```python
from build123d import *

# Parameters (mm, degrees)
SKETCH_W            = 9
SKETCH_H            = 10
PAD_DEPTH           = 30
SKETCH001_R         = 1.5
POCKET_DEPTH        = 5.501
POCKET_DEPTH_BACK   = 5.501
LINEARPATTERN_COUNT = 4
LINEARPATTERN_PITCH = 6.666667


with BuildPart() as part:
    # Sketch → Pad (new body)
    with BuildSketch(Plane.XY):
        Polygon((-5.5, 6), (-5.5, -6), (-1, -6), (-1, -16), (1, -16), (1, -6), (5.5, -6), (5.5, 6), align=None)
        Rectangle(SKETCH_W, SKETCH_H, mode=Mode.SUBTRACT)
    extrude(amount=PAD_DEPTH)

    # Sketch001 → Pocket (cut, two sides)
    with BuildSketch(Plane.YZ) as pocket_sk:
        with Locations((-11, 5)):
            Circle(SKETCH001_R)
    pocket = extrude(amount=-POCKET_DEPTH, mode=Mode.SUBTRACT) + extrude(pocket_sk.sketch, amount=POCKET_DEPTH_BACK, mode=Mode.SUBTRACT)

    # LinearPattern: Pocket ×4
    with Locations(*[(0, 0, i * LINEARPATTERN_PITCH) for i in range(1, LINEARPATTERN_COUNT)]):
        add(pocket, mode=Mode.SUBTRACT)


solid = part.part
```
Read the model definition and answer for the solid it produces. Units are mm, in the model's axes. A direction names the side the tool comes from. Round coordinates to 2 decimals unless told otherwise and drop trailing zeros. Write each loop counter-clockwise with the first axis right and the second up, starting at its lowest first coordinate (ties: lowest second). Pieces come first, ordered by that corner, then holes. Notation, with made-up numbers: M 34.5,49 L 41.5,49 A21 ccw 41.5,72 Z; hole C 50,-4.5 d5. An arc over 180 degrees is marked long. One line per item, written item: value.
Q1. Find section D-D on x = 2.75. Write down the section's boundary in (y, z).
Data:
outline: M -6,0 L -5,0 L -5,30 L -6,30 Z; M 5,0 L 6,0 L 6,30 L 5,30 Z
Q2. Find section B-B on y = -11. Write down the section's boundary in (x, z).
Data:
outline: M -1,0 L 1,0 L 1,3.5 L -1,3.5 Z; M -1,6.5 L 1,6.5 L 1,10.17 L -1,10.17 Z; M -1,13.17 L 1,13.17 L 1,16.83 L -1,16.83 Z; M -1,19.83 L 1,19.83 L 1,23.5 L -1,23.5 Z; M -1,26.5 L 1,26.5 L 1,30 L -1,30 Z
Q3. Find section C-C on z = 14.5. Write down the section's boundary in (x, y).
Data:
outline: M -5.5,-6 L -1,-6 L -1,-16 L 1,-16 L 1,-6 L 5.5,-6 L 5.5,6 L -5.5,6 Z; hole M -4.5,-5 L 4.5,-5 L 4.5,5 L -4.5,5 Z
Q4. Which of the six approach directions +Z, -Z, +X, -X, +Y, -Y give full straight-line access (tool end or side, diameter ignored) to faces 4 (the flat face through (-1, -11, 15)), 5 (the flat face through (-5, -3, 0)), 6 (the flat face through (3, -6, 15)), 7 (the flat face through (-4.5, 0, 15)), 8 (the cylindrical face through (0.014, -12.19, 10.754))?
Data:
face 4: +Z, -Z, -X, -Y
face 5: -Z, +X, -X, +Y, -Y
face 6: +Z, -Z, +X, -Y
face 7: +Z, -Z
face 8: +X, -X
Q5. Straight lines are drawn through the part: line 1 (Z direction, x = 0.5, y = -11); line 2 (X direction, y = -4.5, z = 21.25); line 3 (Y direction, x = 0.1, z = 5). For each, find the intervals that lie inside material, in ascending order. Write a range as [from, to].
Data:
line 1: [0, 3.5], [6.5, 10.17], [13.17, 16.83], [19.83, 23.5], [26.5, 30]
line 2: [-5.5, -4.5], [4.5, 5.5]
line 3: [-16, -12.5], [-9.5, -5], [5, 6]
Q6. For a pull along X with two mould halves and no side action, classify faces 1 (the cylindrical face through (0.014, -12.106, 19.347)), 2 (the flat face through (1, -11, 15)), 3 (the flat face through (4.5, 0, 15)) as +X half, -X half, draft (parallel to the pull), parting line (faces both ways), or undercut.
Data:
face 1: draft
face 2: +X half
face 3: undercut
Q7. Flat-ended cylindrical pins translate along their axes: pin 1 Ø5 at (y, z) = (-9, 11) entering from -X; pin 2 Ø5 at (y, z) = (-11, 5) entering from +X; pin 3 Ø1.3 at (x, z) = (3.5, 21.5) entering from -Y. Find the tip coordinate at first contact, or state that the pin passes through.
Data:
pin 1: x = -1
pin 2: x = 1
pin 3: y = -6
Q8. Find section A-A on z = 5. Write down the section's boundary in (x, y), plus the area to 3 significant figures.
Data:
outline: M -5.5,-6 L -1,-6 L -1,-9.5 L 1,-9.5 L 1,-6 L 5.5,-6 L 5.5,6 L -5.5,6 Z; M -1,-16 L 1,-16 L 1,-12.5 L -1,-12.5 Z; hole M -4.5,-5 L 4.5,-5 L 4.5,5 L -4.5,5 Z
area: 56.0 mm2
